from build123d import *

# Parameters (mm, degrees)
SKETCH1_W           = 100
SKETCH1_H           = 76
BOSS_EXTRUDE1_DEPTH = 5
CUT_EXTRUDE6_REACH  = 7
SKETCH2_R           = 2
SKETCH2_R_2         = 1.832419899


with BuildPart() as part:
    # Sketch1 → Boss-Extrude1 (new body)
    with BuildSketch(Plane(origin=(0, 0, 0), x_dir=(1, 0, 0), z_dir=(0, 1, 0))):
        Rectangle(SKETCH1_W, SKETCH1_H)
    extrude(amount=BOSS_EXTRUDE1_DEPTH)

    # Sketch2 → Cut-Extrude6 (cut, up to next)
    with BuildSketch(Plane(origin=(0, 5, 0), x_dir=(1, 0, 0), z_dir=(0, 1, 0)), mode=Mode.PRIVATE) as cut_extrude6_sk1:
        with Locations((-46, 34)):
            Circle(SKETCH2_R)
    cut_extrude6_tool1 = extrude(cut_extrude6_sk1.sketch, amount=-CUT_EXTRUDE6_REACH, mode=Mode.PRIVATE) & part.part
    add(cut_extrude6_tool1.solids().sort_by_distance((-46, 5, -34))[0], mode=Mode.SUBTRACT)
    # Sketch2 → Cut-Extrude6 (cut, up to next)
    with BuildSketch(Plane(origin=(0, 5, 0), x_dir=(1, 0, 0), z_dir=(0, 1, 0)), mode=Mode.PRIVATE) as cut_extrude6_sk2:
        with Locations((-28, 34)):
            Circle(SKETCH2_R)
    cut_extrude6_tool2 = extrude(cut_extrude6_sk2.sketch, amount=-CUT_EXTRUDE6_REACH, mode=Mode.PRIVATE) & part.part
    add(cut_extrude6_tool2.solids().sort_by_distance((-28, 5, -34))[0], mode=Mode.SUBTRACT)
    # Sketch2 → Cut-Extrude6 (cut, up to next)
    with BuildSketch(Plane(origin=(0, 5, 0), x_dir=(1, 0, 0), z_dir=(0, 1, 0)), mode=Mode.PRIVATE) as cut_extrude6_sk3:
        with Locations((-46, -32)):
            Circle(SKETCH2_R)
    cut_extrude6_tool3 = extrude(cut_extrude6_sk3.sketch, amount=-CUT_EXTRUDE6_REACH, mode=Mode.PRIVATE) & part.part
    add(cut_extrude6_tool3.solids().sort_by_distance((-46, 5, 32))[0], mode=Mode.SUBTRACT)
    # Sketch2 → Cut-Extrude6 (cut, up to next)
    with BuildSketch(Plane(origin=(0, 5, 0), x_dir=(1, 0, 0), z_dir=(0, 1, 0)), mode=Mode.PRIVATE) as cut_extrude6_sk4:
        with Locations((-28, -32)):
            Circle(SKETCH2_R)
    cut_extrude6_tool4 = extrude(cut_extrude6_sk4.sketch, amount=-CUT_EXTRUDE6_REACH, mode=Mode.PRIVATE) & part.part
    add(cut_extrude6_tool4.solids().sort_by_distance((-28, 5, 32))[0], mode=Mode.SUBTRACT)
    # Sketch2 → Cut-Extrude6 (cut, up to next)
    with BuildSketch(Plane(origin=(0, 5, 0), x_dir=(1, 0, 0), z_dir=(0, 1, 0)), mode=Mode.PRIVATE) as cut_extrude6_sk5:
        with Locations((11.2, 27.8)):
            Circle(SKETCH2_R_2)
    cut_extrude6_tool5 = extrude(cut_extrude6_sk5.sketch, amount=-CUT_EXTRUDE6_REACH, mode=Mode.PRIVATE) & part.part
    add(cut_extrude6_tool5.solids().sort_by_distance((11.2, 5, -27.8))[0], mode=Mode.SUBTRACT)
    # Sketch2 → Cut-Extrude6 (cut, up to next)
    with BuildSketch(Plane(origin=(0, 5, 0), x_dir=(1, 0, 0), z_dir=(0, 1, 0)), mode=Mode.PRIVATE) as cut_extrude6_sk6:
        with Locations((43.2, 27.8)):
            Circle(SKETCH2_R_2)
    cut_extrude6_tool6 = extrude(cut_extrude6_sk6.sketch, amount=-CUT_EXTRUDE6_REACH, mode=Mode.PRIVATE) & part.part
    add(cut_extrude6_tool6.solids().sort_by_distance((43.2, 5, -27.8))[0], mode=Mode.SUBTRACT)
    # Sketch2 → Cut-Extrude6 (cut, up to next)
    with BuildSketch(Plane(origin=(0, 5, 0), x_dir=(1, 0, 0), z_dir=(0, 1, 0)), mode=Mode.PRIVATE) as cut_extrude6_sk7:
        with Locations((11.2, -4.2)):
            Circle(SKETCH2_R_2)
    cut_extrude6_tool7 = extrude(cut_extrude6_sk7.sketch, amount=-CUT_EXTRUDE6_REACH, mode=Mode.PRIVATE) & part.part
    add(cut_extrude6_tool7.solids().sort_by_distance((11.2, 5, 4.2))[0], mode=Mode.SUBTRACT)
    # Sketch2 → Cut-Extrude6 (cut, up to next)
    with BuildSketch(Plane(origin=(0, 5, 0), x_dir=(1, 0, 0), z_dir=(0, 1, 0)), mode=Mode.PRIVATE) as cut_extrude6_sk8:
        with Locations((43.2, -4.2)):
            Circle(SKETCH2_R_2)
    cut_extrude6_tool8 = extrude(cut_extrude6_sk8.sketch, amount=-CUT_EXTRUDE6_REACH, mode=Mode.PRIVATE) & part.part
    add(cut_extrude6_tool8.solids().sort_by_distance((43.2, 5, 4.2))[0], mode=Mode.SUBTRACT)


solid = part.part
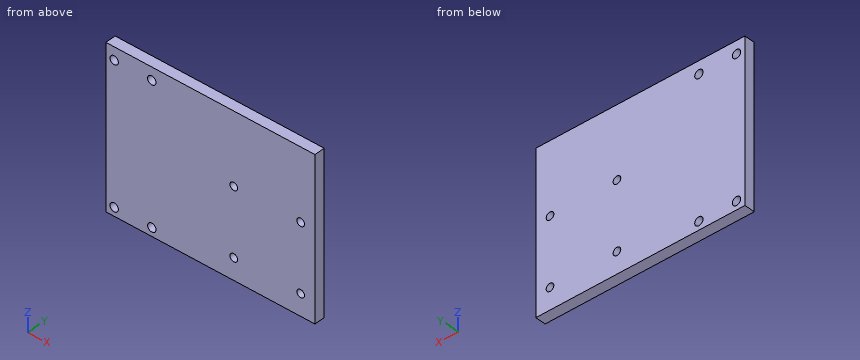
Could you check a few things on this model? Use its own coordinates, in mm. Give positions to 0.01 mm unless a question says otherwise; leave off trailing zeros. Order: outer loops, then holes, each group sorted by start corner. A loop starts at its lowest first (then second) coordinate and runs counter-clockwise, first axis right, second up.
1. Suppose I cut it at A-A (x = 43.2). Write out the boundary of the cut face in (y, z), plus the area to 3 significant figures.
Answers below:
outline: (0, -38) - (5, -38) - (5, -29.63) - (0, -29.63) - close; (0, -25.97) - (5, -25.97) - (5, 2.37) - (0, 2.37) - close; (0, 6.03) - (5, 6.03) - (5, 38) - (0, 38) - close
area: 343 mm2
2. I need wall thicknesses on L1, parallel to X at y = 2.8, z = 4.2; L2, parallel to Z at x = -46, y = 2.6; L3, parallel to X at y = 1.45, z = 32. Which ranges of each line are inside material? Lowest first, please.
Answers below:
L1: x = -50 to 9.37, 13.03 to 41.37, 45.03 to 50
L2: z = -38 to -36, -32 to 30, 34 to 38
L3: x = -50 to -48, -44 to -30, -26 to 50
3. Suppose I cut it at B-B (z = 32). Write out the boundary of the cut face in (x, y), plus the area to 3 significant figures.
Answers below:
outline: (-50, 0) - (-48, 0) - (-48, 5) - (-50, 5) - close; (-44, 0) - (-30, 0) - (-30, 5) - (-44, 5) - close; (-26, 0) - (50, 0) - (50, 5) - (-26, 5) - close
area: 460 mm2
